from build123d import *

# Parameters (mm, degrees)
F0_R     = 32.6029937505
F1_DEPTH = 2.286
F2_R     = 22.8313061555
F3_DEPTH = 1.524
F6_R     = 29.7880355639
F7_DEPTH = 1.016


# Not quite as in the source:
# - a fillet or chamfer that OpenCascade refuses, or shapes differently, is made with other operations: its cross-section is extruded or revolved along the edge and cut away or added


with BuildPart() as f1:
    # F0 (on Right) → F1 (new body)
    with BuildSketch(Plane.YZ):
        with Locations((-40.8581867814, 32.8951068223)):
            Circle(F0_R)
    extrude(amount=F1_DEPTH)

    # F2 (on face) → F3 (join)
    with BuildSketch(Plane.YZ.offset(2.286)):
        with Locations((-40.8581867814, 32.8951068223)):
            Circle(F2_R)
    extrude(amount=F3_DEPTH)

    # F4: fillet of radius 5.08 on 1 edges, made by hand

    # F4_s1 → F4_t2 (revolve, cut)
    with BuildSketch(Plane.XY.offset(32.8951068223)):
        with BuildLine():
            ThreePointArc((2.286, -18.0268806259), (3.4135285843, -19.6872507278), (3.81, -21.6547262676))
            Line((3.81, -21.6547262676), (3.81, -18.0268806259))
            Line((3.81, -18.0268806259), (2.286, -18.0268806259))
        make_face()
    revolve(axis=Axis((3.81, -40.8581867814, 32.8951068223), (1, 0, 0)), mode=Mode.SUBTRACT)

    # F5: fillet of radius 5.08 on 1 edges, made by hand

    # F5_s1 → F5_t2 (revolve, cut)
    with BuildSketch(Plane.XY.offset(32.8951068223)):
        with BuildLine():
            ThreePointArc((0, -8.2551930309), (1.6781314829, -10.0881738983), (2.286, -12.4978294754))
            Line((2.286, -12.4978294754), (2.286, -8.2551930309))
            Line((2.286, -8.2551930309), (0, -8.2551930309))
        make_face()
    revolve(axis=Axis((2.286, -40.8581867814, 32.8951068223), (1, 0, 0)), mode=Mode.SUBTRACT)

    # F6 (on face) → F7 (cut)
    with BuildSketch(Plane(origin=(0, 0, 0), x_dir=(0, -1, 0), z_dir=(-1, 0, 0))):
        with Locations((40.8581867814, 32.8951068223)):
            Circle(F6_R)
    extrude(amount=-F7_DEPTH, mode=Mode.SUBTRACT)

    # F8: fillet of radius 5.08 on 1 edges, made by hand

    # F8_s1 → F8_t2 (revolve)
    with BuildSketch(Plane.XY.offset(32.8951068223)):
        with BuildLine():
            ThreePointArc((0, -70.6462223453), (0.7553111541, -69.2046593967), (1.016, -67.5982223453))
            Line((1.016, -67.5982223453), (1.016, -70.6462223453))
            Line((1.016, -70.6462223453), (0, -70.6462223453))
        make_face()
    revolve(axis=Axis((1.016, -40.8581867814, 32.8951068223), (-1, 0, 0)))


solid = f1.part
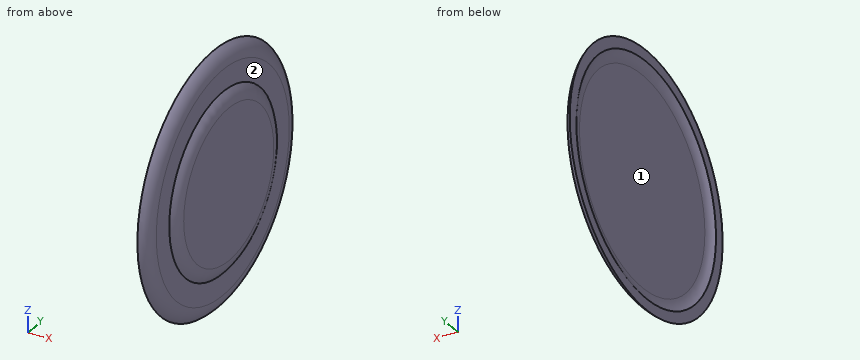
Design review of the part built by this model. Coordinates are the model's own, in mm. Face numbers are marked on the shaded views. Coordinates: 2 decimals unless noted, no trailing zeros. Loops run counter-clockwise (first coordinate to the right, second up) from the corner with the lowest first, then second, coordinate; pieces in that order, holes last. Notation, with made-up numbers: M 88,26.5 L 146,26.5 A27 ccw 146,60.5 Z; hole C 71.5,2.25 d7. An arc over 180 degrees is marked long. Use one line per item in the form item = value.
(1) Draft analysis for pull direction Y (two halves, no side actions). For the marked faces 1 and 2, state which applies: pulls with the +Y half, pulls with the -Y half, needs draft (parallel to the pull), parting line crosses it, or undercut.
Return value:
face_1 = undercut
face_2 = needs draft
(2) Consider section A-A (x = 3). Write out the cut boundary in (y, z).
Return value:
outline = C -40.86,32.9 d43.91
(3) For line 1 along X through (y, z) = (-36, 10); line 2 along Y through (x, z) = (1.4, 49); line 3 along Z through (x, y) = (0.4, -27.5), list the stretches that pass through material, from the lowest coordinate up. Write a range as from..to.
Return value:
line_1 = 1.02..2.29
line_2 = -67.61..-14.1
line_3 = 3.48..6.97, 58.82..62.32
(4) Clearance check with flat-ended pins moving along their axes: P1, Ø1.5, axis at y = -63, z = 22, coming from the +X side; P2, Ø16, axis at y = -49, z = 34.5, coming from the -X side. State where each tip first meets the part, or that it passes through.
Return value:
P1 = 2.29
P2 = 1.02
